The model under review builds one solid part; all positions refer to its coordinate system, in mm. Face numbers are marked on the shaded views. A direction names the side the tool comes from. Round coordinates to 2 decimals unless told otherwise and drop trailing zeros. Write each loop counter-clockwise with the first axis right and the second up, starting at its lowest first coordinate (ties: lowest second). Pieces come first, ordered by that corner, then holes.
Item 1: Add section C-C (x = -1.4). Give the boundary of the cut face in (y, z), plus the area to 3 significant figures.
Item 2: Add section A-A (y = 1). Give the boundary of the cut face in (x, z).
Item 3: Add section B-B (x = 0.85). Give the boundary of the cut face in (y, z).
Item 4: Draft analysis for pull direction X (two halves, no side actions). For the marked faces 3, 4, 5 and 6, state which applies: +X half, -X half, draft (parallel to the pull), parting line (faces both ways), or undercut.
Item 5: Machinability: for the marked faces 1 and 2, which of the approach directions +Z, -Z, +X, -X, +Y, -Y give a long, thin tool a straight path to every point of the face, cutting with its end or side? Answer none if there is none.
Item 6: Add section D-D (y = -1.7). Give the boundary of the cut face in (x, z), plus the area to 3 significant figures.
Item 7: To check wall thickness, follow L1, parallel to Z at x = -0.7, y = -0.05; L2, parallel to Z at x = -1.1, y = -0.05; L3, parallel to X at y = 0.85, z = -0.25. State the ranges of each line that lie inside material, in increasing order.
Item 8: Clearance check with flat-ended pins moving along their axes: pin 1 Ø1 at (y, z) = (0.5, -1.5) entering from +X; pin 2 Ø0.8 at (y, z) = (-0.5, 1) entering from +X; pin 3 Ø1 at (y, z) = (1, -2.5) entering from -X. State where each tip first meets the part, or that it passes through.
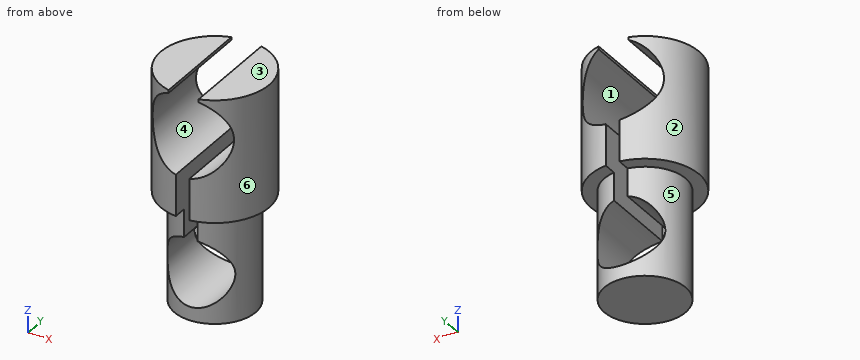
```python
from build123d import *

# Parameters (mm, degrees)
F0_R     = 1.5
F1_DEPTH = 4
F0_R_2   = 2
F2_DEPTH = 4.5
F4_DEPTH = 2.5


with BuildPart() as f1:
    # F0 (on Top) → F1 (new body)
    with BuildSketch(Plane.XY):
        Circle(F0_R)
    extrude(amount=-F1_DEPTH)

    # F0 (on Top) → F2 (join)
    with BuildSketch(Plane.XY):
        Circle(F0_R_2)
        Circle(F0_R, mode=Mode.SUBTRACT)
        Circle(F0_R)
    extrude(amount=F2_DEPTH)

    # F3 (on Front) → F4 (cut, symmetric)
    with BuildSketch(Plane.XZ):
        with BuildLine():
            ThreePointArc((0.25, 1.5209800542), (1.1456439237, 2.0317541634), (1.5, 3))
            ThreePointArc((1.5, 3), (1.2408554332, 3.8427798015), (0.5529629416, 4.3943571943))
            Line((0.5529629416, 4.3943571943), (-0.5529629416, 4.3943571943))
            ThreePointArc((-0.5529629416, 4.3943571943), (-1.4917310142, 2.8427149678), (-0.25, 1.5209800542))
            Line((-0.25, 1.5209800542), (0.25, 1.5209800542))
        make_face()
        with BuildLine():
            Line((-0.5529629416, 4.3943571943), (0.5529629416, 4.3943571943))
            ThreePointArc((0.5529629416, 4.3943571943), (0.2814819786, 4.473352604), (0, 4.5))
            ThreePointArc((0, 4.5), (-0.2814819786, 4.473352604), (-0.5529629416, 4.3943571943))
        make_face()
        with BuildLine():
            ThreePointArc((0, 4.5), (0.2814819786, 4.473352604), (0.5529629416, 4.3943571943))
            Line((0.5529629416, 4.3943571943), (0.5529629416, 4.5))
            Line((0.5529629416, 4.5), (0, 4.5))
        make_face()
        with BuildLine():
            Line((0.25, -1.0252551286), (0.25, 1.5209800542))
            ThreePointArc((0.25, 1.5209800542), (0, 1.5), (-0.25, 1.5209800542))
            Line((-0.25, 1.5209800542), (-0.25, -1.0252551286))
            ThreePointArc((-0.25, -1.0252551286), (0, -1), (0.25, -1.0252551286))
        make_face()
        with BuildLine():
            ThreePointArc((-0.25, 1.5209800542), (0, 1.5), (0.25, 1.5209800542))
            Line((0.25, 1.5209800542), (-0.25, 1.5209800542))
        make_face()
        with BuildLine():
            ThreePointArc((-0.5529629416, 4.3943571943), (-0.2814819786, 4.473352604), (0, 4.5))
            Line((0, 4.5), (-0.5529629416, 4.5))
            Line((-0.5529629416, 4.5), (-0.5529629416, 4.3943571943))
        make_face()
        with BuildLine():
            Line((-0.25, -1.0252551286), (0.25, -1.0252551286))
            ThreePointArc((0.25, -1.0252551286), (0, -1), (-0.25, -1.0252551286))
        make_face()
        with BuildLine():
            ThreePointArc((1.25, -2.25), (0.9682458366, -1.459430585), (0.25, -1.0252551286))
            Line((0.25, -1.0252551286), (-0.25, -1.0252551286))
            ThreePointArc((-0.25, -1.0252551286), (-0.790569415, -3.2182458366), (1.25, -2.25))
        make_face()
    extrude(amount=F4_DEPTH, both=True, mode=Mode.SUBTRACT)


solid = f1.part
```
Numbers:
1. outline: (-1.43, 0) - (-0.54, 0) - (-0.54, -4) - (0.54, -4) - (0.54, 0) - (1.43, 0) - (1.43, 2.46) - (-1.43, 2.46) - close; (-1.43, 3.54) - (1.43, 3.54) - (1.43, 4.5) - (-1.43, 4.5) - close
1. area: 14.1 mm2
2. outline: (-1.73, 0) - (-1.12, 0) - (-1.12, -1.69) arc R1.25 cw to (-0.25, -1.03) - (-0.25, 1.52) arc R1.5 cw to (-0.55, 4.39) - (-0.55, 4.5) - (-1.73, 4.5) - close; (-1.12, -4) - (1.12, -4) - (1.12, -2.81) arc R1.25 cw to (-1.12, -2.81) - close; (0.25, -1.03) arc R1.25 cw to (1.12, -1.69) - (1.12, 0) - (1.73, 0) - (1.73, 4.5) - (0.55, 4.5) - (0.55, 4.39) arc R1.5 cw to (0.25, 1.52) - close
3. outline: (-1.81, 0) - (-1.24, 0) - (-1.24, -1.33) - (1.24, -1.33) - (1.24, 0) - (1.81, 0) - (1.81, 1.76) - (-1.81, 1.76) - close; (-1.81, 4.24) - (1.81, 4.24) - (1.81, 4.5) - (-1.81, 4.5) - close; (-1.24, -4) - (1.24, -4) - (1.24, -3.17) - (-1.24, -3.17) - close
4. face 3: draft
4. face 4: undercut
4. face 5: parting line
4. face 6: +X half
5. face 1: +Y, -Y
5. face 2: +Z, -Z, -X
6. outline: (-1.05, 0) - (-0.25, 0) - (-0.25, 1.52) arc R1.5 cw to (-1.05, 1.93) - close; (-1.05, 4.07) arc R1.5 cw to (-0.55, 4.39) - (-0.55, 4.5) - (-1.05, 4.5) - close; (0.25, 0) - (1.05, 0) - (1.05, 1.93) arc R1.5 cw to (0.25, 1.52) - close; (0.55, 4.39) arc R1.5 cw to (1.05, 4.07) - (1.05, 4.5) - (0.55, 4.5) - close
6. area: 2.94 mm2
7. L1: z = -4 to -3.29, -1.21 to 1.67, 4.33 to 4.5
7. L2: z = -4 to -2.84, -1.66 to 1.98, 4.02 to 4.5
7. L3: x = -1.24 to -0.25, 0.25 to 1.24
8. pin 1: stops at x = 1.5
8. pin 2: stops at x = 2
8. pin 3: stops at x = -1.41
